Here's how the part is built. I have some questions about the finished solid (model axes, mm). Face numbers are marked on the shaded views. A direction names the side the tool comes from. Coordinates: 2 decimals unless noted, no trailing zeros. Order: outer loops, then holes, each group sorted by start corner. A loop starts at its lowest first (then second) coordinate and runs counter-clockwise, first axis right, second up. Notation, with made-up numbers: (73.25, -15) -> (128.25, -15) arc R14 cw to (128.25, 10) -> close; hole circle Ø4 at (-1.5, -23.75). An arc over 180 degrees is marked (long way). One line per item, written item: value. Start each with the question number.
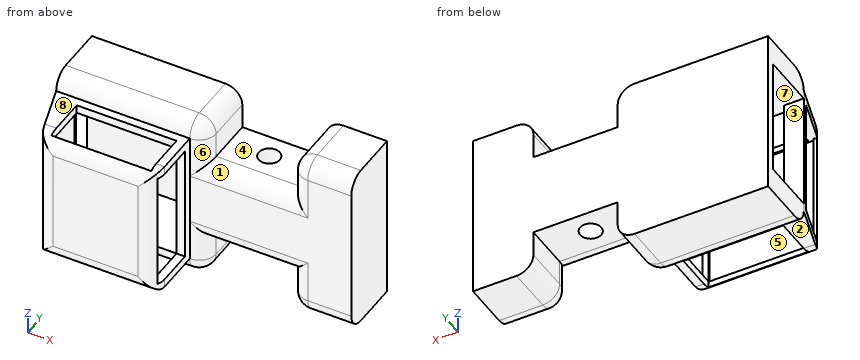
```python
from build123d import *

# Parameters (mm, degrees)
F0_W         = 88.9
F0_H         = 25.4
F1_DEPTH     = 19.05
F2_W         = 25.4
F2_H         = 19.05
F3_DEPTH     = 12.7
F4_R         = 3.175
F5_DEPTH     = 12.7
F7_R         = 5.08
F8_W         = 37.6902104366
F8_H         = 35.56
F9_DEPTH     = 16.51
F10_W        = 40.2302104366
F10_H        = 40.64
F11_DEPTH    = 18.55363
F12_W        = 31.75
F12_H        = 35.56
F13_DEPTH    = 16.51
F14_W        = 30.0702104366
F14_H        = 13.47363
F15_DEPTH    = 2.54
F16_W        = 30.0702104366
F16_H        = 13.47363
F17_DEPTH    = 2.54
F19_DEPTH    = 50.8
F20_W        = 14.3303479189
F20_H        = 35.56
F21_DEPTH    = 7.62
F22_W        = 13.47363
F22_H        = 35.56
F23_DEPTH    = 5.08
F24_T1_DEPTH = 59.4053934524
F24_T3_DEPTH = 59.927191924
F24_T5_DEPTH = 66.04


# Not quite as in the source:
# - a fillet or chamfer that OpenCascade refuses, or shapes differently, is made with other operations: its cross-section is extruded or revolved along the edge and cut away or added


with BuildPart() as f1:
    # F0 (on Front) → F1 (new body)
    with BuildSketch(Plane.XZ):
        with Locations((44.45, 12.7)):
            Rectangle(F0_W, F0_H)
    extrude(amount=F1_DEPTH)

    # F2 (on face) → F3 (cut)
    with BuildSketch(Plane.XY.offset(25.4)):
        with Locations((58.0102104366, -9.525)):
            Rectangle(F2_W, F2_H)
    extrude(amount=-F3_DEPTH, mode=Mode.SUBTRACT)

    # F4 (on face) → F5 (cut)
    with BuildSketch(Plane.XY.offset(12.7)):
        with Locations((57.3752104366, -6.985)):
            Circle(F4_R)
    extrude(amount=-F5_DEPTH, mode=Mode.SUBTRACT)

    # F6: F1 across plane


with BuildPart() as f1_1:
    add(f1.part)
    add(f1.part.mirror(Plane.XY))

    # F7
    f7_edges = [f1_1.edges().sort_by_distance(p)[0] for p in [
        (22.655105, -19.05, -25.4),
        (22.655105, -19.05, 25.4),
        (45.31021, -9.525, -25.4),
        (45.31021, -19.05, -19.05),
        (70.71021, -19.05, -19.05),
        (70.71021, -9.525, -25.4),
        (70.71021, -9.525, 25.4),
        (70.71021, -19.05, 19.05),
        (45.31021, -9.525, 25.4),
        (45.31021, -19.05, 19.05),
        (58.01021, -19.05, -12.7),
        (58.01021, -19.05, 12.7),
        (79.805105, -19.05, -25.4),
        (79.805105, -19.05, 25.4),
    ]]
    fillet(f7_edges, radius=F7_R)

    # F8 (on face) → F9 (cut)
    with BuildSketch(Plane.XZ.offset(19.05)):
        with Locations((18.8451052183, 0)):
            Rectangle(F8_W, F8_H)
    extrude(amount=-F9_DEPTH, mode=Mode.SUBTRACT)

    # F10 (on face) → F11 (join)
    with BuildSketch(Plane.XZ.offset(19.05)):
        with Locations((20.1151052183, 0)):
            Rectangle(F10_W, F10_H)
    extrude(amount=F11_DEPTH)

    # F12 (on face) → F13 (cut)
    with BuildSketch(Plane(origin=(0, -19.05, 0), x_dir=(-1, 0, 0), z_dir=(0, 1, 0))):
        with Locations((-21.8152104366, 0)):
            Rectangle(F12_W, F12_H)
    extrude(amount=-F13_DEPTH, mode=Mode.SUBTRACT)

    # F14 (on face) → F15 (cut)
    with BuildSketch(Plane(origin=(0, 0, -20.32), x_dir=(1, 0, 0), z_dir=(0, 0, -1))):
        with Locations((22.6551052183, 28.326815)):
            Rectangle(F14_W, F14_H)
    extrude(amount=-F15_DEPTH, mode=Mode.SUBTRACT)

    # F16 (on face) → F17 (cut)
    with BuildSketch(Plane.XY.offset(20.32)):
        with Locations((22.6551052183, -28.326815)):
            Rectangle(F16_W, F16_H)
    extrude(amount=-F17_DEPTH, mode=Mode.SUBTRACT)

    # F18 (on face) → F19 (cut)
    with BuildSketch(Plane.XY.offset(20.32)):
        Polygon((0, -37.60363), (5.7030185126, -37.60363), (0, -19.05), align=None)
    extrude(amount=-F19_DEPTH, mode=Mode.SUBTRACT)

    # F20 (on face) → F21 (cut)
    with BuildSketch(Plane(origin=(-5.3501013979, -1.6445152413, 0), x_dir=(0.293813307, -0.9558628252, 0), z_dir=(-0.9558628252, -0.293813307, 0))):
        with Locations((27.9143607796, 0)):
            Rectangle(F20_W, F20_H)
    extrude(amount=-F21_DEPTH, mode=Mode.SUBTRACT)

    # F22 (on face) → F23 (cut)
    with BuildSketch(Plane.YZ.offset(40.2302104366)):
        with Locations((-28.326815, 0)):
            Rectangle(F22_W, F22_H)
    extrude(amount=-F23_DEPTH, mode=Mode.SUBTRACT)

    # F24: fillet of radius 5.08 on 4 edges, made by hand

    # F24_s2 → F24_t1 (cut)
    with BuildSketch(Plane.XY.offset(-29.7026967262)):
        with BuildLine():
            ThreePointArc((9.4560972031, -37.60363), (6.4374769658, -36.6094997805), (4.600314051, -34.0162015997))
            Line((4.600314051, -34.0162015997), (5.7030185126, -37.60363))
            Line((5.7030185126, -37.60363), (9.4560972031, -37.60363))
        make_face()
    extrude(amount=F24_T1_DEPTH, mode=Mode.SUBTRACT)

    # F24_s4 → F24_t3 (cut)
    with BuildSketch(Plane.YZ.offset(-6.9969814874)):
        with BuildLine():
            ThreePointArc((-37.60363, 15.24), (-36.1157324484, 18.8321024484), (-32.52363, 20.32))
            Line((-32.52363, 20.32), (-37.60363, 20.32))
            Line((-37.60363, 20.32), (-37.60363, 15.24))
        make_face()
        with BuildLine():
            ThreePointArc((-37.60363, -15.24), (-36.1157324484, -18.8321024484), (-32.52363, -20.32))
            Line((-32.52363, -20.32), (-37.60363, -20.32))
            Line((-37.60363, -20.32), (-37.60363, -15.24))
        make_face()
    extrude(amount=F24_T3_DEPTH, mode=Mode.SUBTRACT)

    # F24_s6 → F24_t5 (cut)
    with BuildSketch(Plane.XY.offset(-33.02)):
        with BuildLine():
            ThreePointArc((40.2302104366, -32.52363), (38.742312885, -36.1157324484), (35.1502104366, -37.60363))
            Line((35.1502104366, -37.60363), (40.2302104366, -37.60363))
            Line((40.2302104366, -37.60363), (40.2302104366, -32.52363))
        make_face()
    extrude(amount=F24_T5_DEPTH, mode=Mode.SUBTRACT)


solid = f1_1.part
```
Q1. Imagine slicing it at D-D (y = -24). Write out the boundary of the cut face in (x, z), plus the area to 3 significant figures.
Q2. For the marked faces 1, 2, 3, 4 and 5, which set-ups out of +Z, -Z, +X, -X, +Y, -Y let a thin tool reach every point of the face, with its end or its side?
Q3. Imagine slicing it at A-A (x = 17.5). Write out the boundary of the cut face in (y, z), plus the area to 3 significant figures.
Q4. Imagine slicing it at C-C (y = -8). Write out the boundary of the cut face in (x, z).
Q5. If we mould it in two halves opening along Z, with no side actions, what happens to the marked faces 6, 7 and 8? For each: +Z half, -Z half, draft (parallel to the pull), parting line (faces both ways), or undercut.
Q6. Imagine slicing it at B-B (z = -9). Write out the boundary of the cut face in (x, y) (3 decimals).
Q7. For P1, Ø1.3, axis at y = -31.5, z = -19, coming from the +X side; P2, Ø4, axis at x = 63.5, y = -8, coming from the +Z side; P3, Ø5, axis at y = -11, z = -4, coming from the -X side, each with a flat end and sliding along its axis, tell me the tip position at first contact or that it passes through.
Q8. I need wall thicknesses on line 1 (X direction, y = -8.5, z = 18.5); line 2 (Y direction, x = 31, z = 15); line 3 (Z direction, x = 15.5, y = -14). Which ranges of each line are inside material? Lowest first, please.
Completed:
1. outline: (1.52, -20.32) -> (7.62, -20.32) -> (7.62, -17.78) -> (1.52, -17.78) -> close; (1.52, 17.78) -> (7.62, 17.78) -> (7.62, 20.32) -> (1.52, 20.32) -> close; (37.69, -20.32) -> (40.23, -20.32) -> (40.23, -17.78) -> (37.69, -17.78) -> close; (37.69, 17.78) -> (40.23, 17.78) -> (40.23, 20.32) -> (37.69, 20.32) -> close
1. area: 43.9 mm2
2. face 1: +Z, -Y
2. face 2: -Z, +X, -X, -Y
2. face 3: -X
2. face 4: +Z, +Y, -Y
2. face 5: none
3. outline: (-37.6, -15.24) arc R5.08 ccw to (-35.06, -19.64) -> (-35.06, -17.78) -> (-35.56, -17.78) -> (-35.56, 17.78) -> (-35.06, 17.78) -> (-35.06, 19.64) arc R5.08 ccw to (-37.6, 15.24) -> close; (-21.59, -20.32) -> (-19.05, -20.32) arc R5.08 ccw to (-13.97, -25.4) -> (0, -25.4) -> (0, 25.4) -> (-13.97, 25.4) arc R5.08 ccw to (-19.05, 20.32) -> (-21.59, 20.32) -> (-21.59, 17.78) -> (-2.54, 17.78) -> (-2.54, -17.78) -> (-21.59, -17.78) -> close
3. area: 458 mm2
4. outline: (0, -25.4) -> (40.23, -25.4) arc R5.08 ccw to (45.31, -20.32) -> (45.31, -12.7) -> (54.37, -12.7) -> (54.37, 12.7) -> (45.31, 12.7) -> (45.31, 20.32) arc R5.08 ccw to (40.23, 25.4) -> (0, 25.4) -> (0, 17.78) -> (37.69, 17.78) -> (37.69, -17.78) -> (0, -17.78) -> close; (60.38, -12.7) -> (70.71, -12.7) -> (70.71, -20.32) arc R5.08 ccw to (75.79, -25.4) -> (88.9, -25.4) -> (88.9, 25.4) -> (75.79, 25.4) arc R5.08 ccw to (70.71, 20.32) -> (70.71, 12.7) -> (60.38, 12.7) -> close
5. face 6: draft
5. face 7: undercut
5. face 8: +Z half
6. outline: (0, -19.05) -> (0.746, -21.478) -> (5.94, -19.881) -> (5.94, -19.05) -> close; (0, -2.54) -> (37.69, -2.54) -> (37.69, -21.59) -> (40.23, -21.59) -> (40.23, -19.05) arc R5.08 ccw to (41.61, -18.859) -> (74.41, -18.859) arc R5.08 ccw to (75.79, -19.05) -> (88.9, -19.05) -> (88.9, 0) -> (0, 0) -> close; (5.097, -35.133) arc R5.08 ccw to (9.456, -37.604) -> (35.15, -37.604) arc R5.08 ccw to (39.55, -35.064) -> (37.69, -35.064) -> (37.69, -35.56) -> (5.94, -35.56) -> (5.94, -34.873) -> close; hole circle Ø6.35 at (57.375, -6.985)
7. P1: stops at x = 40.23
7. P2: stops at z = 12.7
7. P3: stops at x = 37.69
8. line 1: x = 0 to 45.31, 70.71 to 88.9
8. line 2: y = -37.6 to -35.56, -2.54 to 0
8. line 3: z = -25.4 to -17.78, 17.78 to 25.4
